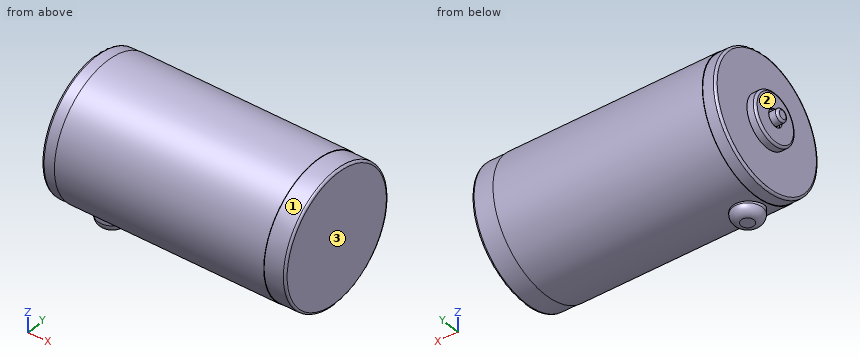
```python
from build123d import *

# Parameters (mm, degrees)
SKETCH007_R  = 3.5
PAD004_DEPTH = 18
FILLET_R     = 2
FILLET001_R  = 0.5


with BuildPart() as part:
    # Sketch006 → Revolution (revolve)
    with BuildSketch(Plane.XY):
        Polygon((-38.2, 0), (-38.2, 15.5), (-43.2, 15.5), (-43.2, 15.6), (-92.2, 15.6), (-92.2, 15.5), (-95.2, 15.5), (-95.2, 6), (-97.2, 6), (-97.2, 2), (-96.7, 2), (-96.7, 1.5), (-98.9, 1.5), (-98.9, 0), align=None)
    revolve(axis=Axis((0, 0, 0), (1, 0, 0)))

    # Sketch007 → Pad004 (new body)
    with BuildSketch(Plane.XY):
        with Locations((-88, -3.5)):
            Circle(SKETCH007_R)
    extrude(amount=-PAD004_DEPTH)

    # Fillet
    fillet_edges = [part.edges().sort_by_distance(p)[0] for p in [
        (-91.5, -3.5, -18),
    ]]
    fillet(fillet_edges, radius=FILLET_R)

    # Fillet001
    fillet001_edges = [part.edges().sort_by_distance(p)[0] for p in [
        (-95.2, -15.5, 0),
        (-38.2, -15.5, 0),
        (-97.2, -6, 0),
        (-98.9, -1.5, 0),
    ]]
    fillet(fillet001_edges, radius=FILLET001_R)


with BuildPart() as part_1:
    # Body001 placement: moved
    add(part.part.moved(Location((0, -0.5, -17.9))))


solid = part_1.part
```
Can you work these out from the model? Positions are in its coordinate system, mm. Face numbers are marked on the shaded views. A direction names the side the tool comes from. Coordinates: 2 decimals unless noted, no trailing zeros. Write each loop counter-clockwise with the first axis right and the second up, starting at its lowest first coordinate (ties: lowest second). Pieces come first, ordered by that corner, then holes. Notation, with made-up numbers: M 39,38 L 44,38 A20 cw 44,74 Z; hole C 68,27.25 d4. An arc over 180 degrees is marked long. Answer as CSV lines item,"result".
Item 1: I'm going to push flat-ended pins straight in: P1, Ø6, axis at x = -71, z = -29.5, coming from the -Y side; P2, Ø2, axis at x = -76, y = 10, coming from the +Z side; P3, Ø6, axis at x = -59.5, y = 4, coming from the +Z side. Where does each tip first touch, or does it pass through?
Geometry results:
P1,"stops at y = -13.52"
P2,"stops at z = -5.53"
P3,"stops at z = -2.37"
Item 2: Imagine slicing it at B-B on x = -41.5. List the corners of the cut face in (y, z) for me, plus the area to 3 significant figures.
Geometry results:
outline,"C -0.5,-17.9 d31"
area,"755 mm2"
Item 3: Please list where these lines run through material, in increasing order: line 1 along Z through (x, y) = (-96.9, -0.5); line 2 along Z through (x, y) = (-97.1, -0.5); line 3 along X through (y, z) = (8, -30).
Geometry results:
line 1,"z = -23.86 to -19.9, -19.4 to -16.4, -15.9 to -11.94"
line 2,"z = -23.7 to -19.9, -19.4 to -16.4, -15.9 to -12.1"
line 3,"x = -95.2 to -38.2"
Item 4: Imagine slicing it at C-C on x = -65. List the corners of the cut face in (y, z) for me.
Geometry results:
outline,"C -0.5,-17.9 d31.2"
Item 5: On a 3-axis mill with a long thin cutter (end or side, diameter ignored), from which of +Z, -Z, +X, -X, +Y, -Y can I reach the whole of each face in a straight line? I mean the marked faces 1, 2 and 3. Say none if no direction works.
Geometry results:
face 1,"+X"
face 2,"-X"
face 3,"+Z, -Z, +X, +Y, -Y"
